Autodesk Inventor part; units mm, degrees
ref_plane "YZ Plane" through (0, 0, 0) normal (1, 0, 0) x (0, 1, 0)
ref_plane "XZ Plane" through (0, 0, 0) normal (0, 1, 0) x (-1, 0, 0)
ref_plane "XY Plane" through (0, 0, 0) normal (0, 0, 1) x (1, 0, 0)
sketch "Sketch3" plane through (0, 0, 0) normal (0, 0, 1) x (1, 0, 0)
  line L0 (0, 0) -> (16, 0)
  line L1 (16, 0) -> (16, 20)
  line L2 (16, 20) -> (0, 20)
  line L3 (0, 20) -> (0, 0)
  dimension "d0" = 16
  dimension "d1" = 20
extrude "Extrusion1" add sketch "Sketch3" along normal blind 16
fillet "Fillet1" radius 7 2 edges at (16, 10, 16) (0, 10, 16)
fillet "Fillet2" radius 5 2 edges at (16, 10, 0) (0, 10, 0)
sketch "Sketch4" plane through (16, 0, 9) normal (1, 0, 0) x (0, 0, -1)
  line L0 (4, 20) -> (0, 20)
  line L1 (4, 20) -> (-7, 13.6491)
  line L2 (-7, 20) -> (-7, 0)
  line L3 (4, 20) -> (16.7017, 20) construction
  line L4 (-7, 13.6491) -> (-7, 20)
  line L5 (-7, 20) -> (4, 20)
  line L6 (4, 0) -> (0, 0)
  line L7 (4, 0) -> (-7, 6.3509)
  line L8 (4, 0) -> (16.7017, 0) construction
  line L9 (-7, 6.3509) -> (-7, 0)
  line L10 (-7, 0) -> (4, 0)
  point P0 (9, 0)
  point P1 (-7, 0)
  point P2 (0, 0)
  dimension "d6" = 150
  dimension "d7" = 150
extrude "Extrusion2" cut sketch "Sketch4" against normal through all
sketch "Sketch5" plane through (5, 20, 0) normal (0, 1, 0) x (1, 0, 0)
  line L0 (-5, -9) -> (-5, -5)
  line L1 (0, 0) -> (6, 0)
  line L2 (5, 0) -> (1, 0)
  line L3 (1, 0) -> (1, -5)
  line L4 (1, -5) -> (5, -5)
  line L5 (5, -5) -> (5, 0)
  line L6 (1, 0) -> (5, 0)
  point P0 (-5, 0)
  dimension "d47" = 4
extrude "Extrusion3" add sketch "Sketch5" along normal blind 6
sketch "Sketch11" plane through (0, 0, 0) normal (0, 0, -1) x (-1, 0, 0)
  line L0 (-11, 0) -> (-11, 20)
  line L1 (-9, 13.6491) -> (-9, 6.3509)
  line L2 (-11, 0) -> (-9, 0)
  line L3 (-9, 0) -> (-9, 7)
  line L4 (-9, 7) -> (-11, 7)
  line L5 (-11, 7) -> (-11, 0)
  line L6 (-5, 0) -> (-7, 0)
  line L7 (-7, 0) -> (-7, 7)
  line L8 (-7, 7) -> (-5, 7)
  line L9 (-5, 7) -> (-5, 0)
  line L10 (-11, 20) -> (-9, 20)
  line L11 (-9, 20) -> (-9, 13)
  line L12 (-9, 13) -> (-11, 13)
  line L13 (-11, 13) -> (-11, 20)
  line L14 (-5, 20) -> (-7, 20)
  line L15 (-7, 20) -> (-7, 13)
  line L16 (-7, 13) -> (-5, 13)
  line L17 (-5, 13) -> (-5, 20)
  point P0 (0, 0)
  point P1 (-9, 6.3509)
  point P2 (-11, 13)
  dimension "d32" = 7
  dimension "d33" = 2
  dimension "d34" = 7
  dimension "d35" = 7
  dimension "d36" = 7
extrude "Extrusion9" add sketch "Sketch11" along normal blind 3 contours L0 L4 L1 L3 L2 | L0 L10 L11 L1 L12 | L6 L7 L8 L9 | L17 L16 L15 L14
sketch "Sketch12" plane through (0, 0, -3) normal (0, 0, -1) x (-1, 0, 0)
  line L0 (-9, 20) -> (-11, 20)
  line L1 (-5, 13) -> (-7, 13)
  line L2 (-11, 20) -> (-5, 20)
  line L3 (-5, 20) -> (-5, 13)
  line L4 (-5, 13) -> (-11, 13)
  line L5 (-11, 13) -> (-11, 20)
  line L6 (-11, 0) -> (-16, 0)
  line L7 (-11, 0) -> (-5, 0)
  line L8 (-5, 0) -> (-5, 7.0241)
  line L9 (-5, 7.0241) -> (-11, 7.0241)
  line L10 (-11, 7.0241) -> (-11, 0)
  point P0 (0, 0)
  point P1 (-5, -20)
  point P2 (-11, -13)
extrude "Extrusion10" add sketch "Sketch12" along normal blind 2
sketch "Sketch13" plane through (0, 0, 5) normal (0, -1, 0) x (1, 0, 0)
  circle A0 centre (8, 2.5) radius 0.75
  point P0 (0, -5)
  dimension "d42" = 1.5
extrude "Extrusion11" cut sketch "Sketch13" against normal through all
fillet "Fillet4" radius 2 4 edges at (11, 16.5, -5) (5, 16.5, -5) (5, 3.5121, -5) (11, 3.5121, -5)
sketch "Sketch14" plane through (10, 20, 5) normal (1, 0, 0) x (0, 0, -1)
  circle A0 centre (2.5, 3.5) radius 2.025
  line L0 (0, 6) -> (5, 6)
  point P0 (5, -20)
  dimension "d48" = 4.05
  dimension "d59" = 2.5
extrude "Extrusion12" cut sketch "Sketch14" against normal blind 5
sketch "Sketch15" plane through (0, 0, 5) normal (0, -1, 0) x (1, 0, 0)
  line L0 (10, -5) -> (10, 0)
  line L1 (10, 0) -> (6, 0)
  line L2 (6, 0) -> (6, -5)
  line L3 (6, -5) -> (10, -5)
  line L4 (10, -5) -> (10, 0)
  point P0 (0, -5)
  point P1 (10, -0.475)
  point P2 (6, -0.475)
  dimension "d60" = 5
  dimension "d61" = 4
extrude "Extrusion13" add sketch "Sketch15" along normal blind 6
sketch "Sketch16" plane through (10, 0, 5) normal (1, 0, 0) x (0, 0, -1)
  circle A0 centre (2.5, -3.5) radius 2.025
  line L0 (5, -6) -> (0, -6)
  point P0 (5, 0)
  dimension "d54" = 4.05
  dimension "d58" = 2.5
extrude "Extrusion14" cut sketch "Sketch16" against normal blind 5
fillet "Fillet7" radius 1 1 edges at (8, -6, 5)
sketch "Sketch17" plane through (0, -6, 5) normal (0, -1, 0) x (1, 0, 0)
  line L0 (6, -5) -> (10, -5)
  line L1 (6, -4.525) -> (6, -0.475)
  line L2 (10, -5) -> (6, -5)
  line L3 (6, -5) -> (6, -2)
  line L4 (6, -2) -> (10, -2)
  line L5 (10, -2) -> (10, -5)
  point P0 (0, -5)
  point P1 (6, -5)
  dimension "d63" = 3
extrude "Extrusion15" add sketch "Sketch17" along normal blind 1
fillet "Fillet8" radius 1 1 edges at (8, 26, 5)
sketch "Sketch18" plane through (5, 26, 0) normal (0, 1, 0) x (1, 0, 0)
  line L0 (1, -3) -> (5, -3)
  line L1 (1, -5) -> (1, 0)
  line L2 (5, -3) -> (1, -3)
  line L3 (1, -3) -> (1, 0)
  line L4 (1, 0) -> (5, 0)
  line L5 (5, 0) -> (5, -3)
  point P0 (-5, 0)
extrude "Extrusion16" add sketch "Sketch18" along normal blind 1
sketch "Sketch19" plane through (6, 0, 0) normal (-1, 0, 0) x (0, 0, 1)
  line L0 (3, -6) -> (3, -7)
  line L1 (0, 0) -> (0, -7)
  line L2 (3, -6) -> (0, -7)
  line L3 (0, -7) -> (3, -7)
  line L4 (3, -7) -> (3, -6)
extrude "Extrusion17" cut sketch "Sketch19" against normal through all
sketch "Sketch20" plane through (6, 20, 0) normal (-1, 0, 0) x (0, 0, 1)
  line L0 (4, 6) -> (3, 6)
  line L1 (0, 0) -> (0, 7)
  line L2 (3, 6) -> (0, 7)
  line L3 (0, 7) -> (3, 7)
  line L4 (3, 7) -> (3, 6)
  point P0 (0, -20)
extrude "Extrusion18" cut sketch "Sketch20" against normal through all
sketch "Sketch22" plane through (16, 0, 5) normal (1, 0, 0) x (0, 0, -1)
  point P0 (5, 0)
sketch "Sketch23" plane through (16, 0, 5) normal (1, 0, 0) x (0, 0, -1)
  line L0 (0, 0) -> (-4, 2.3094)
  line L1 (-4, 2.3094) -> (-11, 6.3509)
  line L2 (0, 0) -> (-8.6603, 0)
  line L3 (-8.6603, 0) -> (-8.6603, 5)
  line L4 (-8.6603, 5) -> (0, 5)
  line L5 (0, 5) -> (0, 0)
  point P0 (5, 0)
  dimension "d75" = 5
extrude "Extrusion20" cut sketch "Sketch23" against normal through all contours L0 L1 L4 L5
properties part number "FingerMiddle"
The model under review builds one solid part; all positions refer to its coordinate system, in mm. A direction names the side the tool comes from. Round coordinates to 2 decimals unless told otherwise and drop trailing zeros. Loops run counter-clockwise (first coordinate to the right, second up) from the corner with the lowest first, then second, coordinate; pieces in that order, holes last. Notation, with made-up numbers: (-16.75, 37.25) -> (11.25, 37.25) arc R9 cw to (11.25, 50.25) -> close; hole circle Ø2 at (23, 29.5). An arc over 180 degrees is marked (long way). One line per question, with ' | ' between items. Start each with the question number.
Item 1: Add section D-D, the plane y = 3. Write out the cut boundary in (x, z), then the cut area to 3 significant figures.
Item 2: Wall thickness on line 1 along Y through (x, z) = (9, 2.5) (3 decimals); line 2 along X through (y, z) = (16.25, 7.5); line 3 along Y through (x, z) = (4, 3.25): over which ranges is each line inside the solid? List them lowest first. Write a range as [from, to].
Item 3: Draft analysis for pull direction X (two halves, no side actions). For faces 5 (the face through (5, 4, -1)), 6 (the face through (8, 26.5, 1.5)), 7 (the face through (7, 17, -1)), state which applies: +X half, -X half, draft (parallel to the pull), parting line (faces both ways), or undercut.
Item 4: Add section B-B, the plane y = 23.5. Write out the cut boundary in (x, z) (3 decimals), then the cut area to 3 significant figures.
Item 5: For pin 1 (1.5 mm diameter, centred on y = 5, z = -1.5, fed in from -X); pin 2 (8 mm diameter, centred on x = 5.5, z = 8, fed in from +Y); pin 3 (1.5 mm diameter, centred on x = 8.5, z = -1, fed in from +Y); pin 4 (4 mm diameter, centred on y = 2, z = 8, fed in from -X) (3 decimals), all flat-tipped, find the tip position at first contact; note any pin that passes through.
Item 6: Add section A-A, the plane z = -1.75. Write out the cut boundary in (x, y).
Item 7: Machinability: for faces 1 (the face through (8, 10, 0)), 2 (the face through (8, -6, 3.5)), 3 (the face through (10, 21, 2)), 4 (the face through (10, -1, 3)), which of the approach directions +Z, -Z, +X, -X, +Y, -Y give a long, thin tool a straight path to every point of the face, cutting with its end or side? Answer none if there is none.
Item 8: Add section C-C, the plane x = 8. Write out the cut boundary in (y, z) (3 decimals).
Return value:
1) outline: (0, 5) arc R5 ccw to (5, 0) -> (5, -3) arc R2 ccw to (7, -5) -> (9, -5) arc R2 ccw to (11, -3) -> (11, 0) arc R5 ccw to (16, 5) -> close; hole (7, -3) -> (9, -3) -> (9, 0) -> (7, 0) -> close | area: 91.6 mm2
2) line 1: y = [-6.167, -5.525], [-1.475, 21.475], [25.525, 26.167] | line 2: x = [0, 7.25], [8.75, 16] | line 3: y = [0, 20]
3) face 5: -X half | face 6: draft | face 7: undercut
4) outline: (6, 0) -> (10, 0) -> (10, 0.475) -> (6, 0.475) -> close; (6, 4.525) -> (10, 4.525) -> (10, 5) -> (6, 5) -> close | area: 3.80 mm2
5) pin 1: stops at x = 5 | pin 2: stops at y = 26 | pin 3: stops at y = 20 | pin 4: passes through
6) outline: (5, 0) -> (7, 0) -> (7, 7) -> (5, 7) -> close; (5, 13) -> (7, 13) -> (7, 20) -> (5, 20) -> close; (9, 0) -> (11, 0) -> (11, 7) -> (9, 7) -> close; (9, 13) -> (11, 13) -> (11, 20) -> (9, 20) -> close
7) face 1: none | face 2: +Z, +X, -X, -Y | face 3: +Z, -Z, +X, +Y | face 4: +Z, -Z, +X, -Y
8) outline: (-7, 0) -> (27, 0) -> (26, 3) -> (26, 4) arc R1 ccw to (25, 5) -> (20, 5) -> (18.99, 6.75) -> (5, 6.75) -> (5, 5) -> (-5, 5) arc R1 ccw to (-6, 4) -> (-6, 3) -> close; (0, -5) -> (7.024, -5) -> (7.024, -3) -> (0, -3) -> close; (5, 8.25) -> (18.124, 8.25) -> (13.649, 16) -> (6.351, 16) -> (5, 13.66) -> close; (13, -5) -> (20, -5) -> (20, -3) -> (13, -3) -> close; hole circle Ø4.05 at (-3.5, 2.5); hole circle Ø4.05 at (23.5, 2.5)
